CAD build for the part. Positions are in the model's coordinates, mm. Give positions to 0.01 mm unless a question says otherwise; leave off trailing zeros. Loops run counter-clockwise (first coordinate to the right, second up) from the corner with the lowest first, then second, coordinate; pieces in that order, holes last.
Item 1: Mould opens along Z. For faces 1 (the cylindrical face through (20.05, 1.58, -0.13)), 2 (the conical face through (16.1, 0.81, 1.07)), 3 (the flat face through (0, 2, -6)), 4 (the flat face through (0, 0, -3)) say: released by +Z, released by -Z, zero draft, split by the parting line, or undercut.
Item 2: Probe probe 1 along X at (y, z) = (0.4, 0); probe 2 along X at (y, z) = (0.9, -0.5); probe 3 along Z at (x, y) = (0, 0.55). List the from-to ranges inside material, lowest first.
Item 3: Saw through at B-B on z = 0. Give the cut face in (x, y), plus the area to 3 significant figures.
Item 4: Saw through at D-D on z = -1.5. Give the number of separate pieces and of enclosed holes in the cut face, plus the area to 3 significant figures.
Item 5: Saw through at A-A on y = 1.4. Give the cut face in (x, z), plus the area to 3 significant figures.
Item 6: Drop a flat-ended pin along its axis: P1, Ø1, axis at y = 1, z = -3.5, coming from the -X side. Give the stop position or say it passes through.
Item 7: Saw through at C-C on x = 0. Give the cut face in (y, z).
from build123d import *

# Parameters (mm, degrees)
BOSS_EXTRUDE2_DEPTH                          = 3.2
CSK_FOR_M4_COUNTERSUNK_FLAT_HEAD1_AT_2_COUNT = 2
CSK_FOR_M4_COUNTERSUNK_FLAT_HEAD1_AT_2_PITCH = 14.05
CSK_FOR_M4_COUNTERSUNK_FLAT_HEAD1_AT_3_COUNT = 2
CSK_FOR_M4_COUNTERSUNK_FLAT_HEAD1_AT_3_PITCH = 14.05


with BuildPart() as part:
    # Sketch3 → Boss-Extrude2 (new body)
    with BuildSketch(Plane(origin=(0, 0, 0), x_dir=(1, 0, 0), z_dir=(0, 1, 0))):
        with BuildLine():
            Line((-14.05, 6), (14.05, 6))
            ThreePointArc((14.05, 6), (20.05, 0), (14.05, -6))
            Line((14.05, -6), (-14.05, -6))
            ThreePointArc((-14.05, -6), (-20.05, 0), (-14.05, 6))
        make_face()
    extrude(amount=BOSS_EXTRUDE2_DEPTH)

    # Sketch5 → CSK for M4 Countersunk Flat Head1 (revolve, cut)
    with BuildSketch(Plane(origin=(0, 3.2, 0), x_dir=(0, 0, 1), z_dir=(1, 0, 0))):
        Polygon((0, 0), (0, 3.2), (2.15, 3.2), (2.15, 2.55), (4.7, 0), align=None)
    csk_for_m4_countersunk_flat_head1 = revolve(axis=Axis((0, 9.55, 0), (0, -1, 0)), mode=Mode.SUBTRACT)

    # CSK for M4 Countersunk Flat Head1 at 2: CSK for M4 Countersunk Flat Head1 ×2
    with Locations(*[(i * CSK_FOR_M4_COUNTERSUNK_FLAT_HEAD1_AT_2_PITCH, 0, 0) for i in range(1, CSK_FOR_M4_COUNTERSUNK_FLAT_HEAD1_AT_2_COUNT)]):
        add(csk_for_m4_countersunk_flat_head1, mode=Mode.SUBTRACT)

    # CSK for M4 Countersunk Flat Head1 at 3: CSK for M4 Countersunk Flat Head1 ×2
    with Locations(*[(-i * CSK_FOR_M4_COUNTERSUNK_FLAT_HEAD1_AT_3_PITCH, 0, 0) for i in range(1, CSK_FOR_M4_COUNTERSUNK_FLAT_HEAD1_AT_3_COUNT)]):
        add(csk_for_m4_countersunk_flat_head1, mode=Mode.SUBTRACT)


solid = part.part
Results below:
1. face 1: split by the parting line
1. face 2: undercut
1. face 3: released by -Z
1. face 4: zero draft
2. probe 1: x = -20.05 to -16.2, -11.9 to -2.15, 2.15 to 11.9, 16.2 to 20.05
2. probe 2: x = -20.03 to -16.4, -11.7 to -2.35, 2.35 to 11.7, 16.4 to 20.03
2. probe 3: z = -6 to -2.15, 2.15 to 6
3. outline: (-20.05, 0) - (-16.2, 0) - (-16.2, 0.65) - (-18.75, 3.2) - (-20.05, 3.2) - close; (-11.9, 0) - (-2.15, 0) - (-2.15, 0.65) - (-4.7, 3.2) - (-9.35, 3.2) - (-11.9, 0.65) - close; (2.15, 0) - (11.9, 0) - (11.9, 0.65) - (9.35, 3.2) - (4.7, 3.2) - (2.15, 0.65) - close; (16.2, 0) - (20.05, 0) - (20.05, 3.2) - (18.75, 3.2) - (16.2, 0.65) - close
3. area: 67.5 mm2
4. separate pieces: 4
4. enclosed holes: 0
4. area: 74.4 mm2
5. outline: (-14.05, -6) - (14.05, -6) arc R6 ccw to (14.05, 6) - (-14.05, 6) arc R6 ccw to start; hole circle Ø5.8 at (-14.05, 0); hole circle Ø5.8 at (0, 0); hole circle Ø5.8 at (14.05, 0)
5. area: 371 mm2
6. P1: stops at x = -19.25
7. outline: (0, -6) - (3.2, -6) - (3.2, -4.7) - (0.65, -2.15) - (0, -2.15) - close; (0, 2.15) - (0.65, 2.15) - (3.2, 4.7) - (3.2, 6) - (0, 6) - close
